The listing builds one solid part. Answer for the finished solid, in the listing's coordinates (mm). Face numbers are marked on the shaded views. A direction names the side the tool comes from. Coordinates: 2 decimals unless noted, no trailing zeros. Order: outer loops, then holes, each group sorted by start corner. A loop starts at its lowest first (then second) coordinate and runs counter-clockwise, first axis right, second up. Notation, with made-up numbers: (0.25, 46) -> (20.25, 46) arc R16 cw to (20.25, 76) -> close; hole circle Ø2 at (0, 36.25). An arc over 180 degrees is marked (long way). Answer in a Markdown table with one row per item.
```python
from build123d import *

# Parameters (mm, degrees)
SKETCH1_R           = 7.5
BOSS_EXTRUDE1_DEPTH = 8
SKETCH2_R           = 12.7
BOSS_EXTRUDE2_DEPTH = 12.7
CHAMFER1_SIZE       = 1.27
CUT_EXTRUDE2_DEPTH  = 12.7


with BuildPart() as part:
    # Sketch1 → Boss-Extrude1 (new body)
    with BuildSketch(Plane.XY):
        Circle(SKETCH1_R)
        with BuildLine():
            Line((-2.711977876, 1.651), (2.711977876, 1.651))
            ThreePointArc((2.711977876, 1.651), (0, -3.175), (-2.711977876, 1.651))
        make_face(mode=Mode.SUBTRACT)
    extrude(amount=BOSS_EXTRUDE1_DEPTH)

    # Sketch2 → Boss-Extrude2 (add)
    with BuildSketch(Plane.XY.offset(8)):
        Circle(SKETCH2_R)
    extrude(amount=BOSS_EXTRUDE2_DEPTH)

    # Chamfer1
    chamfer1_edges = [part.edges().sort_by_distance(p)[0] for p in [
        (-12.7, 0, 8),
        (-12.7, 0, 20.7),
    ]]
    chamfer(chamfer1_edges, length=CHAMFER1_SIZE)

    # Sketch3 → Cut-Extrude2 (cut)
    with BuildSketch(Plane.XY.offset(20.7)):
        with BuildLine():
            Line((-1.494578623, 13.823081897), (-0.508, 11.418705531))
            ThreePointArc((-0.508, 11.418705531), (0, 11.43), (0.508, 11.418705531))
            Line((0.508, 11.418705531), (1.494578623, 13.823081897))
            Line((1.494578623, 13.823081897), (-1.494578623, 13.823081897))
        make_face()
        with BuildLine():
            Line((3.909053826, 13.342812918), (6.670675026, 12.198911963))
            Line((6.670675026, 12.198911963), (4.839080228, 10.355105144))
            ThreePointArc((4.839080228, 10.355105144), (4.374071632, 10.559943057), (3.900418623, 10.743911511))
            Line((3.900418623, 10.743911511), (3.909053826, 13.342812918))
        make_face()
        with BuildLine():
            Line((8.717568266, 10.831221626), (10.831221626, 8.717568266))
            Line((10.831221626, 8.717568266), (8.433454358, 7.715033868))
            ThreePointArc((8.433454358, 7.715033868), (8.082230509, 8.082230509), (7.715033868, 8.433454358))
            Line((7.715033868, 8.433454358), (8.717568266, 10.831221626))
        make_face()
        with BuildLine():
            Line((12.198911963, 6.670675026), (13.342812918, 3.909053826))
            Line((13.342812918, 3.909053826), (10.743911511, 3.900418623))
            ThreePointArc((10.743911511, 3.900418623), (10.559943057, 4.374071632), (10.355105144, 4.839080228))
            Line((10.355105144, 4.839080228), (12.198911963, 6.670675026))
        make_face()
        with BuildLine():
            Line((13.823081897, 1.494578623), (13.823081897, -1.494578623))
            Line((13.823081897, -1.494578623), (11.418705531, -0.508))
            ThreePointArc((11.418705531, -0.508), (11.43, 0), (11.418705531, 0.508))
            Line((11.418705531, 0.508), (13.823081897, 1.494578623))
        make_face()
        with BuildLine():
            Line((13.342812918, -3.909053826), (12.198911963, -6.670675026))
            Line((12.198911963, -6.670675026), (10.355105144, -4.839080228))
            ThreePointArc((10.355105144, -4.839080228), (10.559943057, -4.374071632), (10.743911511, -3.900418623))
            Line((10.743911511, -3.900418623), (13.342812918, -3.909053826))
        make_face()
        with BuildLine():
            Line((10.831221626, -8.717568266), (8.717568266, -10.831221626))
            Line((8.717568266, -10.831221626), (7.715033868, -8.433454358))
            ThreePointArc((7.715033868, -8.433454358), (8.082230509, -8.082230509), (8.433454358, -7.715033868))
            Line((8.433454358, -7.715033868), (10.831221626, -8.717568266))
        make_face()
        with BuildLine():
            Line((6.670675026, -12.198911963), (3.909053826, -13.342812918))
            Line((3.909053826, -13.342812918), (3.900418623, -10.743911511))
            ThreePointArc((3.900418623, -10.743911511), (4.374071632, -10.559943057), (4.839080228, -10.355105144))
            Line((4.839080228, -10.355105144), (6.670675026, -12.198911963))
        make_face()
        with BuildLine():
            Line((1.494578623, -13.823081897), (-1.494578623, -13.823081897))
            Line((-1.494578623, -13.823081897), (-0.508, -11.418705531))
            ThreePointArc((-0.508, -11.418705531), (0, -11.43), (0.508, -11.418705531))
            Line((0.508, -11.418705531), (1.494578623, -13.823081897))
        make_face()
        with BuildLine():
            Line((-3.909053826, -13.342812918), (-6.670675026, -12.198911963))
            Line((-6.670675026, -12.198911963), (-4.839080228, -10.355105144))
            ThreePointArc((-4.839080228, -10.355105144), (-4.374071632, -10.559943057), (-3.900418623, -10.743911511))
            Line((-3.900418623, -10.743911511), (-3.909053826, -13.342812918))
        make_face()
        with BuildLine():
            Line((-8.717568266, -10.831221626), (-10.831221626, -8.717568266))
            Line((-10.831221626, -8.717568266), (-8.433454358, -7.715033868))
            ThreePointArc((-8.433454358, -7.715033868), (-8.082230509, -8.082230509), (-7.715033868, -8.433454358))
            Line((-7.715033868, -8.433454358), (-8.717568266, -10.831221626))
        make_face()
        with BuildLine():
            Line((-12.198911963, -6.670675026), (-13.342812918, -3.909053826))
            Line((-13.342812918, -3.909053826), (-10.743911511, -3.900418623))
            ThreePointArc((-10.743911511, -3.900418623), (-10.559943057, -4.374071632), (-10.355105144, -4.839080228))
            Line((-10.355105144, -4.839080228), (-12.198911963, -6.670675026))
        make_face()
        with BuildLine():
            Line((-13.823081897, -1.494578623), (-13.823081897, 1.494578623))
            Line((-13.823081897, 1.494578623), (-11.418705531, 0.508))
            ThreePointArc((-11.418705531, 0.508), (-11.43, 0), (-11.418705531, -0.508))
            Line((-11.418705531, -0.508), (-13.823081897, -1.494578623))
        make_face()
        with BuildLine():
            Line((-13.342812918, 3.909053826), (-12.198911963, 6.670675026))
            Line((-12.198911963, 6.670675026), (-10.355105144, 4.839080228))
            ThreePointArc((-10.355105144, 4.839080228), (-10.559943057, 4.374071632), (-10.743911511, 3.900418623))
            Line((-10.743911511, 3.900418623), (-13.342812918, 3.909053826))
        make_face()
        with BuildLine():
            Line((-10.831221626, 8.717568266), (-8.717568266, 10.831221626))
            Line((-8.717568266, 10.831221626), (-7.715033868, 8.433454358))
            ThreePointArc((-7.715033868, 8.433454358), (-8.082230509, 8.082230509), (-8.433454358, 7.715033868))
            Line((-8.433454358, 7.715033868), (-10.831221626, 8.717568266))
        make_face()
        with BuildLine():
            Line((-6.670675026, 12.198911963), (-3.909053826, 13.342812918))
            Line((-3.909053826, 13.342812918), (-3.900418623, 10.743911511))
            ThreePointArc((-3.900418623, 10.743911511), (-4.374071632, 10.559943057), (-4.839080228, 10.355105144))
            Line((-4.839080228, 10.355105144), (-6.670675026, 12.198911963))
        make_face()
    extrude(amount=-CUT_EXTRUDE2_DEPTH, mode=Mode.SUBTRACT)


solid = part.part
```
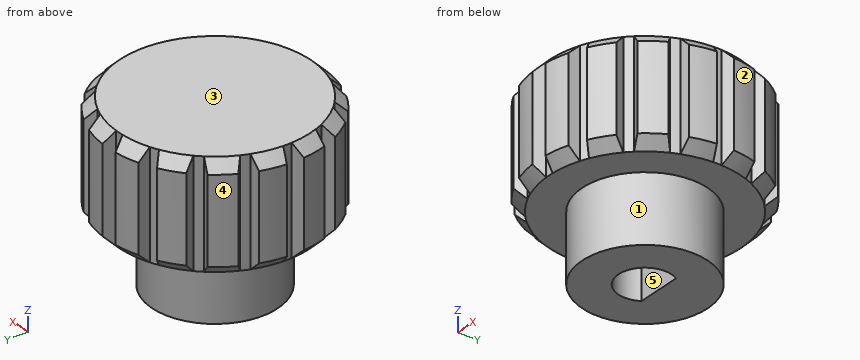
(1) Flat-ended cylindrical pins translate along their axes: pin 1 (12 mm diameter, centred on x = 0.5, y = 7.5, fed in from -Z); pin 2 (8 mm diameter, centred on y = -8, z = 14.5, fed in from +X); pin 3 (1.6 mm diameter, centred on x = 0.5, z = 6, fed in from -Y); pin 4 (3 mm diameter, centred on y = -5, z = 11.5, fed in from +X). Find the tip coordinate at first contact, or state that the pin passes through.
Check values:
| item | result |
|---|---|
| pin 1 | z = 0 |
| pin 2 | x = 11.31 |
| pin 3 | y = -7.5 |
| pin 4 | x = 12.21 |
(2) A cutting plane is placed at B-B, the plane y = 0. Determine the outline of the cut face in (x, z) (3 decimals), then the cut area to 3 significant figures.
Check values:
| item | result |
|---|---|
| outline | (-11.43, 8) -> (-7.5, 8) -> (-7.5, 0) -> (-3.175, 0) -> (-3.175, 8) -> (3.175, 8) -> (3.175, 0) -> (7.5, 0) -> (7.5, 8) -> (11.43, 8) -> (11.43, 20.7) -> (-11.43, 20.7) -> close |
| area | 360 mm² |
(3) Which of the six approach directions +Z, -Z, +X, -X, +Y, -Y give full straight-line access (tool end or side, diameter ignored) to the marked faces 1 and 2?
Check values:
| item | result |
|---|---|
| face 1 | -Z |
| face 2 | +Z, -Z, +X, +Y |
(4) A cutting plane is placed at C-C, the plane z = 4.75. Determine the outline of the cut face in (x, y) (3 decimals).
Check values:
| item | result |
|---|---|
| outline | circle Ø15 at (0, 0); hole (-2.712, 1.651) arc R3.175 ccw (long way) to (2.712, 1.651) -> close |
(5) A cutting plane is placed at A-A, the plane x = 0. Determine the outline of the cut face in (y, z) (3 decimals), then the cut area to 3 significant figures.
Check values:
| item | result |
|---|---|
| outline | (-11.43, 8) -> (-7.5, 8) -> (-7.5, 0) -> (-3.175, 0) -> (-3.175, 8) -> (1.651, 8) -> (1.651, 0) -> (7.5, 0) -> (7.5, 8) -> (11.43, 8) -> (11.43, 20.7) -> (-11.43, 20.7) -> close |
| area | 372 mm² |
(6) For a pull along X with two mould halves and no side action, classify the marked faces 3, 4 and 5 as released by +X, released by -X, zero draft, split by the parting line, or undercut.
Check values:
| item | result |
|---|---|
| face 3 | zero draft |
| face 4 | released by -X |
| face 5 | undercut |
(7) Find the intervals of material crossed by line 1 along Y through (x, z) = (0, 2) (3 decimals); line 2 along Y through (x, z) = (11, 18.5); line 3 along X through (y, z) = (0.25, 15), in increasing order. Write a range as from..to.
Check values:
| item | result |
|---|---|
| line 1 | -7.5..-3.175, 1.651..7.5 |
| line 2 | -6.35..-5.48, -3.9..3.9, 5.48..6.35 |
| line 3 | -11.43..11.43 |
